Autodesk Inventor part; units mm, degrees
ref_plane "YZ Plane" through (0, 0, 0) normal (1, 0, 0) x (0, 1, 0)
ref_plane "XZ Plane" through (0, 0, 0) normal (0, 1, 0) x (-1, 0, 0)
ref_plane "XY Plane" through (0, 0, 0) normal (0, 0, 1) x (1, 0, 0)
sketch "Sketch1" plane through (0, 0, 0) normal (0, 0, 1) x (1, 0, 0)
  line L0 (0, 70) -> (0, -70)
  line L1 (-70, 0) -> (70, 0)
  line L2 (-50, 50) -> (50, 50)
  line L3 (50, 50) -> (50, -50)
  line L4 (50, -50) -> (-50, -50)
  line L5 (-50, -50) -> (-50, 50)
  circle A0 centre (0, 0) radius 30
  dimension "d0" = 100
  dimension "d1" = 100
  dimension "d2" = 60
extrude "Extrusion1" add sketch "Sketch1" along normal blind 20 contours L2 L3 L1 A0 L0 | L0 A0 L1 L5 L2 | L1 L3 L4 L0 A0 | A0 L0 L4 L5 L1
sketch "Sketch2" plane through (-50, -50, 0) normal (0, -1, 0) x (1, 0, 0)
  line L0 (20, 20) -> (20, 0)
  line L1 (0, 0) -> (100, 0)
  line L2 (100, 0) -> (100, 20)
  line L3 (0, 20) -> (100, 20)
  line L4 (0, 0) -> (0, 20)
  line L5 (80, 20) -> (80, 0)
  line L6 (0, 0) -> (0, 20)
  line L7 (0, 10) -> (100, 10)
  line L8 (0, 14) -> (100, 14)
  line L9 (0, 6) -> (100, 6)
  point P0 (50, 0)
  dimension "d5" = 4
  dimension "d6" = 4
extrude "Extrusion2" cut sketch "Sketch2" against normal blind 4 contours L3 L5 L8 L0 | L0 L8 L4 L3 | L3 L2 L8 L5 | L9 L5 L1 L0 | L0 L1 L4 L9 | L9 L2 L1 L5
sketch "Sketch3" plane through (0, 0, 0) normal (0, 0, -1) x (-1, 0, 0)
  line L0 (0, -70) -> (0, 70)
  line L1 (0.5, -70) -> (0.5, 70)
  line L2 (-0.5, -70) -> (-0.5, 70)
  line L3 (-50, -46) -> (50, -46)
  line L4 (50, 50) -> (50, -46)
  line L5 (-50, 50) -> (50, 50)
  line L6 (-50, -46) -> (-50, 50)
  circle A0 centre (0, 0) radius 30
  point P0 (0.5, 29.9958)
  point P1 (0.5, 50)
  point P2 (-0.5, 50)
  point P3 (-0.5, 29.9958)
  dimension "d9" = 0.5
  dimension "d10" = 0.5
extrude "Extrusion3" cut sketch "Sketch3" against normal through all contours A0 L2 L5 L0 | L0 L5 L1 A0
sketch "Sketch4" plane through (50, 50, 20) normal (1, 0, 0) x (0, 0, -1)
  line L0 (20, 0) -> (0, 0)
  line L1 (20, -96) -> (20, 0)
  point P0 (20, -50)
  point P1 (10, -10)
  dimension "d13" = 10
  dimension "d14" = 10
hole "Hole1" at (50, 40, 10) direction (-1, 0, 0) diameter 6.647 depth 110 tip angle 118
sketch "Sketch5" plane through (-50, -50, 14) normal (0, -1, 0) x (1, 0, 0)
  line L0 (100, -14) -> (0, -14)
  line L1 (100, -8) -> (100, 0)
  point P0 (50, -14)
  point P1 (90, -4)
  dimension "d22" = 10
  dimension "d23" = 10
hole "Hole2" at (40, -50, 10) direction (0, 1, 0) diameter 6.647 depth 30 tip angle 118
sketch "Sketch6" plane through (-50, -50, 14) normal (0, -1, 0) x (1, 0, 0)
  line L0 (0, -8) -> (0, 0)
  line L1 (100, -14) -> (0, -14)
  point P0 (50, -14)
  point P1 (10, -4)
  dimension "d31" = 10
  dimension "d32" = 10
hole "Hole3" at (-40, -50, 10) direction (0, 1, 0) diameter 6.647 depth 30 tip angle 118
properties part number "upperClamp"
Part model, mm, in its own coordinate system. A direction names the side the tool comes from. Round coordinates to 2 decimals unless told otherwise and drop trailing zeros. Order: outer loops, then holes, each group sorted by start corner. A loop starts at its lowest first (then second) coordinate and runs counter-clockwise, first axis right, second up. Notation, with made-up numbers: M -7,83 L 29,83 A23 cw 29,113 Z; hole C -29.5,46.5 d3. An arc over 180 degrees is marked long. Put each result on its own line as item: value. Start each with the question number.
1. Slice it at B-B on y = 40. List the corners of the cut face in (x, z).
2. Slice it at D-D on y = -22.5. List the corners of the cut face in (x, z), then the cut area to 3 significant figures.
3. Two-plate mould, pull along X, no slides. Class faces 4 (the face through (-50, -1, 10)), 5 (the face through (-37.05, -34.79, 8.47)), 6 (the face through (-1, -48, 6)), 7 (the face through (-0.5, 40, 5)): +X half, -X half, draft (parallel to the pull), parting line (faces both ways), or undercut.
4. Tool access for faces 1 (the face through (-1, -46, 17)), 2 (the face through (41.27, -34.79, 6.93)), 3 (the face through (0.5, 40, 5)): list every direction of +Z, -Z, +X, -X, +Y, -Y with a clear straight run to the whole face (end or side of a thin tool).
5. Slice it at A-A on x = 24. List the corners of the cut face in (y, z).
6. Drill centre lines: probe 1 along Z at (x, y) = (38, 40); probe 2 along Y at (x, z) = (-44.5, 10); probe 3 along X at (y, z) = (42.5, 5). Where is each one in solid material? Low to high. Write a range as [from, to].
7. Drop flat-ended pins along their axis: pin 1 (1.2 mm diameter, centred on x = -20, y = -48.5, fed in from +Z); pin 2 (5.5 mm diameter, centred on y = 40, z = 10, fed in from -X); pin 3 (1.8 mm diameter, centred on x = -5, z = 2.5, fed in from -Y); pin 4 (4 mm diameter, centred on x = -40, z = 10, fed in from -Y). Give the stop position or say it passes through.
8. Slice it at C-C on z = 18.25. List the corners of the cut face in (x, y), then the cut area to 3 significant figures.
Findings:
1. outline: M -50,0 L -0.5,0 L -0.5,6.68 L -50,6.68 Z; M -50,13.32 L -0.5,13.32 L -0.5,20 L -50,20 Z; M 0.5,0 L 50,0 L 50,6.68 L 0.5,6.68 Z; M 0.5,13.32 L 50,13.32 L 50,20 L 0.5,20 Z
2. outline: M -50,0 L -19.84,0 L -19.84,20 L -50,20 Z; M 19.84,0 L 50,0 L 50,20 L 19.84,20 Z; hole C -40,10 d6.65; hole C 40,10 d6.65
2. area: 1,140 mm2
3. face 4: -X half
3. face 5: undercut
3. face 6: draft
3. face 7: undercut
4. face 1: +Z, +X, -X, -Y
4. face 2: -Y
4. face 3: +Z, -Z, +Y
5. outline: M -50,6 L -46,6 L -46,0 L -18,0 L -18,20 L -46,20 L -46,14 L -50,14 Z; M 18,0 L 50,0 L 50,20 L 18,20 Z; hole C 40,10 d6.65
6. probe 1: [0, 6.68], [13.32, 20]
6. probe 2: [-50, 36.68], [43.32, 50]
6. probe 3: [-50, -0.5], [0.5, 50]
7. pin 1: z = 14
7. pin 2: through
7. pin 3: y = -46
7. pin 4: y = -19.2
8. outline: M -50,-46 L 50,-46 L 50,50 L 0.5,50 L 0.5,30 A30 cw long -0.5,30 L -0.5,50 L -50,50 Z
8. area: 6,750 mm2
